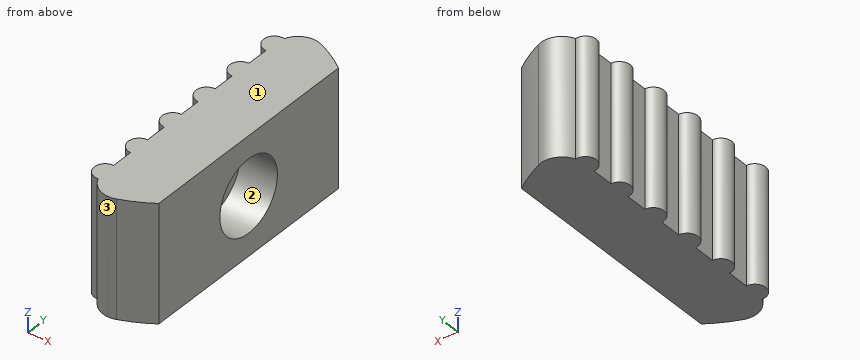
from build123d import *

# Parameters (mm, degrees)
CYLINDER022_R     = 0.5
CYLINDER022_DEPTH = 5.5
CYLINDER020_R     = 0.5
CYLINDER020_DEPTH = 5.5
CYLINDER021_R     = 0.5
CYLINDER021_DEPTH = 5.5
CYLINDER023_R     = 0.5
CYLINDER023_DEPTH = 5.5
CYLINDER018_R     = 0.5
CYLINDER018_DEPTH = 5.5
CYLINDER017_R     = 1.7
CYLINDER017_DEPTH = 10
BOX012_W          = 10
BOX012_H          = 19
BOX012_DEPTH      = 10
BOX015_W          = 10
BOX015_H          = 19
BOX015_DEPTH      = 10
CYLINDER013_R     = 6.5
CYLINDER013_DEPTH = 5.5
FILLET003_R       = 1
CYLINDER024_R     = 0.5
CYLINDER024_DEPTH = 5.5


with BuildPart() as cylinder022:
    # Cylinder022 → Cylinder022 (new body)
    with BuildSketch(Plane(origin=(1, 31, 6.25), x_dir=(1, 0, 0), z_dir=(0, 0, 1))):
        Circle(CYLINDER022_R)
    extrude(amount=CYLINDER022_DEPTH)


with BuildPart() as cylinder020:
    # Cylinder020 → Cylinder020 (new body)
    with BuildSketch(Plane(origin=(1, 35, 6.25), x_dir=(1, 0, 0), z_dir=(0, 0, 1))):
        Circle(CYLINDER020_R)
    extrude(amount=CYLINDER020_DEPTH)


with BuildPart() as cylinder021:
    # Cylinder021 → Cylinder021 (new body)
    with BuildSketch(Plane(origin=(1, 37, 6.25), x_dir=(1, 0, 0), z_dir=(0, 0, 1))):
        Circle(CYLINDER021_R)
    extrude(amount=CYLINDER021_DEPTH)


with BuildPart() as cylinder023:
    # Cylinder023 → Cylinder023 (new body)
    with BuildSketch(Plane(origin=(1, 29, 6.25), x_dir=(1, 0, 0), z_dir=(0, 0, 1))):
        Circle(CYLINDER023_R)
    extrude(amount=CYLINDER023_DEPTH)


with BuildPart() as cylinder018:
    # Cylinder018 → Cylinder018 (new body)
    with BuildSketch(Plane(origin=(1, 27, 6.25), x_dir=(1, 0, 0), z_dir=(0, 0, 1))):
        Circle(CYLINDER018_R)
    extrude(amount=CYLINDER018_DEPTH)


with BuildPart() as cylinder017:
    # Cylinder017 → Cylinder017 (new body)
    with BuildSketch(Plane(origin=(2, 32, 9), x_dir=(0, 0, -1), z_dir=(1, 0, 0))):
        Circle(CYLINDER017_R)
    extrude(amount=CYLINDER017_DEPTH)


with BuildPart() as cube012:
    # Box012 → Box012 (new body)
    with BuildSketch(Plane(origin=(-9, 20.75, 2.25), x_dir=(1, 0, 0), z_dir=(0, 0, 1))):
        with Locations((5, 9.5)):
            Rectangle(BOX012_W, BOX012_H)
    extrude(amount=BOX012_DEPTH)


with BuildPart() as cube015:
    # Box015 → Box015 (new body)
    with BuildSketch(Plane(origin=(3.75, 20.75, 2.25), x_dir=(1, 0, 0), z_dir=(0, 0, 1))):
        with Locations((5, 9.5)):
            Rectangle(BOX015_W, BOX015_H)
    extrude(amount=BOX015_DEPTH)


with BuildPart() as cut002008023012009006003002006_body:
    # Cylinder013 → Cylinder013 (new body)
    with BuildSketch(Plane(origin=(0, 32, 6.25), x_dir=(1, 0, 0), z_dir=(0, 0, 1))):
        Circle(CYLINDER013_R)
    extrude(amount=CYLINDER013_DEPTH)

    # Cut002008023012009006003002006002006002004006: cut Cube015
    add(cube015.part, mode=Mode.SUBTRACT)

    # Cut002008023012009006003002006002006002004007: cut Cube012
    add(cube012.part, mode=Mode.SUBTRACT)

    # Fillet003
    fillet003_edges = [cut002008023012009006003002006_body.edges().sort_by_distance(p)[0] for p in [
        (1, 38.422616, 9),
        (1, 25.577384, 9),
    ]]
    fillet(fillet003_edges, radius=FILLET003_R)

    # Cut002008023012009006003002006002006002004008: cut Cylinder017
    add(cylinder017.part, mode=Mode.SUBTRACT)


with BuildPart() as wire_clamp:
    # Cylinder024 → Cylinder024 (new body)
    with BuildSketch(Plane(origin=(1, 33, 6.25), x_dir=(1, 0, 0), z_dir=(0, 0, 1))):
        Circle(CYLINDER024_R)
    extrude(amount=CYLINDER024_DEPTH)

    # Fusion001001001011002: union Cylinder022, Cylinder020, Cylinder021, Cylinder023, Cylinder018, Cut002008023012009006003002006 body
    add(cylinder022.part)
    add(cylinder020.part)
    add(cylinder021.part)
    add(cylinder023.part)
    add(cylinder018.part)
    add(cut002008023012009006003002006_body.part)


solid = wire_clamp.part
CAD build for the part. Positions are in the model's coordinates, mm. Face numbers are marked on the shaded views. Give positions to 0.01 mm unless a question says otherwise; leave off trailing zeros. Loops run counter-clockwise (first coordinate to the right, second up) from the corner with the lowest first, then second, coordinate; pieces in that order, holes last. Notation, with made-up numbers: M 2,-5 L 22,-5 A16 ccw 22,6 Z; hole C 45.25,3 d5. An arc over 180 degrees is marked long. One line per question, with ' | ' between items. Start each with the question number.
1. Saw through at C-C on y = 32. Give the cut face in (x, z).
2. Two-plate mould, pull along Y, no slides. Class the marked faces 1, 2 and 3: pulls with the +Y half, pulls with the -Y half, needs draft (parallel to the pull), parting line crosses it, or undercut.
3. Flat gauge pins, fed straight in: pin 1 (1 mm diameter, centred on y = 31.5, z = 9, fed in from +X); pin 2 (0.8 mm diameter, centred on y = 28, z = 9.5, fed in from -X). Where does each tip first touch, or does it go through?
4. Saw through at B-B on z = 7. Give the cut face in (x, y), plus the area to 3 significant figures.
5. Saw through at A-A on x = 0.85. Give the cut face in (y, z).
6. Probe L1, parallel to Z at x = 3.25, y = 32; L2, parallel to Y at x = 0.8, z = 8.2; L3, parallel to X at y = 28, z = 7. List the from-to ranges inside material, lowest first. Write a range as from..to.
7. Saw through at D-D on z = 8.25. Give the cut face in (x, y).
Result sheet:
1) outline: M 1,6.25 L 3.75,6.25 L 3.75,7.3 L 2,7.3 L 2,10.7 L 3.75,10.7 L 3.75,11.75 L 1,11.75 Z
2) face 1: needs draft | face 2: undercut | face 3: pulls with the -Y half
3) pin 1: stops at x = 2 | pin 2: stops at x = 1
4) outline: M 1,27.5 A0.5 ccw long 1.07,26.51 A1 ccw 2.36,25.94 A6.5 ccw 3.75,26.69 L 3.75,37.31 A6.5 ccw 2.36,38.06 A1 ccw 1.07,37.49 A0.5 ccw long 1,36.5 L 1,35.5 A0.5 ccw 1,34.5 L 1,33.5 A0.5 ccw 1,32.5 L 1,31.5 A0.5 ccw 1,30.5 L 1,29.5 A0.5 ccw 1,28.5 Z | area: 34.5 mm^2
5) outline: M 26.52,6.25 L 27.48,6.25 L 27.48,11.75 L 26.52,11.75 Z; M 28.52,6.25 L 29.48,6.25 L 29.48,11.75 L 28.52,11.75 Z; M 30.52,6.25 L 31.48,6.25 L 31.48,11.75 L 30.52,11.75 Z; M 32.52,6.25 L 33.48,6.25 L 33.48,11.75 L 32.52,11.75 Z; M 34.52,6.25 L 35.48,6.25 L 35.48,11.75 L 34.52,11.75 Z; M 36.52,6.25 L 37.48,6.25 L 37.48,11.75 L 36.52,11.75 Z
6) L1: z = 6.25..7.3, 10.7..11.75 | L2: y = 26.54..27.46, 28.54..29.46, 30.54..31.46, 32.54..33.46, 34.54..35.46, 36.54..37.46 | L3: x = 1..3.75
7) outline: M 1,27.5 A0.5 ccw long 1.07,26.51 A1 ccw 2.36,25.94 A6.5 ccw 3.75,26.69 L 3.75,30.47 L 2,30.47 L 2,33.53 L 3.75,33.53 L 3.75,37.31 A6.5 ccw 2.36,38.06 A1 ccw 1.07,37.49 A0.5 ccw long 1,36.5 L 1,35.5 A0.5 ccw 1,34.5 L 1,33.5 A0.5 ccw 1,32.5 L 1,31.5 A0.5 ccw 1,30.5 L 1,29.5 A0.5 ccw 1,28.5 Z
